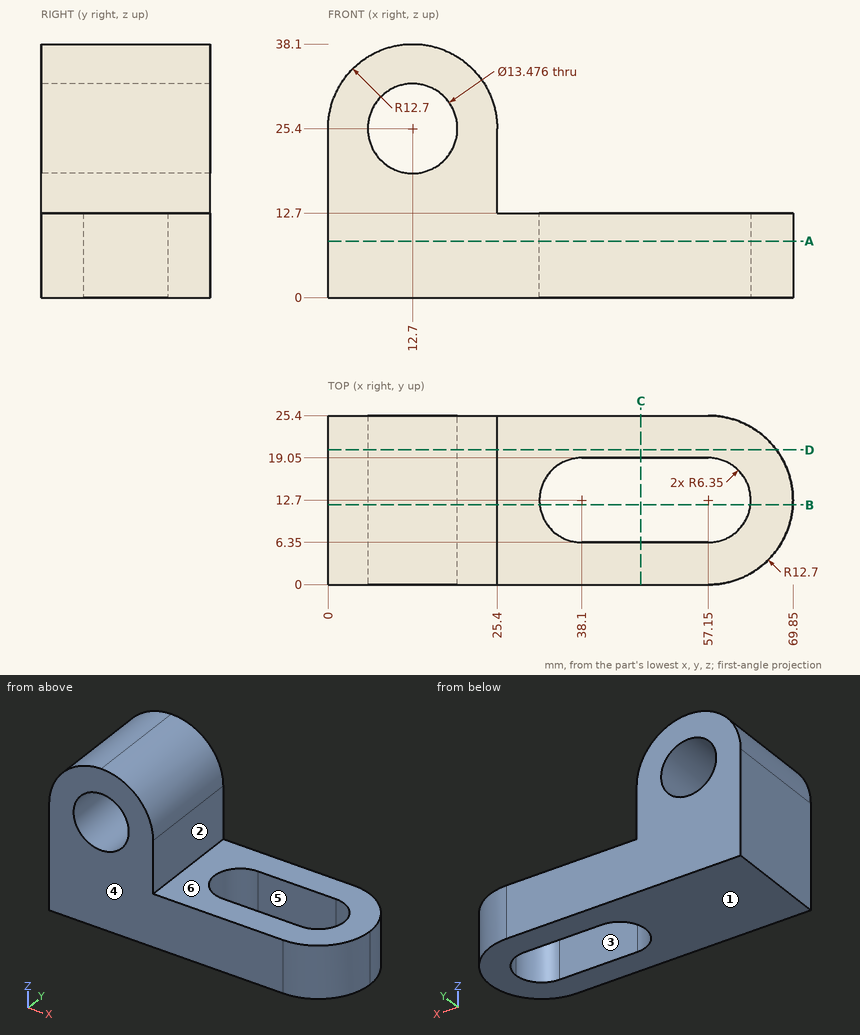
Input: dimensioned drawing with shaded views. Units: mm. Origin: part minimum x, y, z. A direction names the side the tool comes from. Coordinates: 2 decimals unless noted, no trailing zeros. Write each loop counter-clockwise with the first axis right and the second up, starting at its lowest first coordinate (ties: lowest second). Pieces come first, ordered by that corner, then holes. Notation, with made-up numbers: M 61,59.25 L 115,59.25 A26 cw 115,89.25 Z; hole C 31.25,85 d5. An arc over 180 degrees is marked long. Use one line per item in the form item = value.
Q1. Section B-B (y = 12). Return loops of the section in (x, z).
Answer below:
outline = M 0,0 L 31.79,0 L 31.79,12.7 L 25.4,12.7 L 25.4,25.4 A12.7 ccw 0,25.4 Z; M 63.46,0 L 69.83,0 L 69.83,12.7 L 63.46,12.7 Z; hole C 12.7,25.4 d13.48
Q2. Draft query along Y for the marked faces 4, 5 and 6. Return one class per face: released by +Y, released by -Y, zero draft, split by the parting line, or undercut.
Answer below:
face_4 = released by -Y
face_5 = undercut
face_6 = zero draft
Q3. Section D-D (y = 20.25). Return loops of the section in (x, z), plus the area to 3 significant figures.
Answer below:
outline = M 0,0 L 67.36,0 L 67.36,12.7 L 25.4,12.7 L 25.4,25.4 A12.7 ccw 0,25.4 Z; hole C 12.7,25.4 d13.48
area = 1,290 mm²
Q4. Section C-C (x = 47). Return loops of the section in (y, z), plus the area to 3 significant figures.
Answer below:
outline = M 0,0 L 6.35,0 L 6.35,12.7 L 0,12.7 Z; M 19.05,0 L 25.4,0 L 25.4,12.7 L 19.05,12.7 Z
area = 161 mm²
Q5. Set-up query: the marked faces 1, 2 and 3. Return all of +Z, -Z, +X, -X, +Y, -Y with unobstructed straight access to the full face (end or side cutting, diameter ignored); none if empty.
Answer below:
face_1 = -Z, +X, -X, +Y, -Y
face_2 = +Z, +X, +Y, -Y
face_3 = +Z, -Z
Q6. First-contact query: pin 1 (5 mm diameter, centred on x = 35, y = 20, fed in from +Z); pin 2 (6.5 mm diameter, centred on x = 44, z = 8, fed in from -Y); pin 3 (10 mm diameter, centred on y = 11.5, z = 19, fed in from +X). Flat tips, straight axial feed; report the tip coordinate or a pass-through.
Answer below:
pin_1 = 12.7
pin_2 = 0
pin_3 = 25.4
Q7. Section A-A (z = 8.5). Return loops of the section in (x, y).
Answer below:
outline = M 0,0 L 57.15,0 A12.7 ccw 57.15,25.4 L 0,25.4 Z; hole M 38.1,6.35 L 57.15,6.35 A6.35 ccw 57.15,19.05 L 38.1,19.05 A6.35 ccw Z
Q8. Material intervals for probe 1 along X at (y, z) = (12.25, 2.5); probe 2 along Z at (x, y) = (12.7, 7.5); probe 3 along X at (y, z) = (11, 10) (1 decimal), sorted ascending. Write a range as from..to.
Answer below:
probe_1 = 0..31.77, 63.48..69.84
probe_2 = 0..18.66, 32.14..38.1
probe_3 = 0..32, 63.3..69.7
